Geometry check sheet. Reference: the model listing, model coordinates, mm. Give positions to 0.01 mm unless a question says otherwise; leave off trailing zeros. Loops run counter-clockwise (first coordinate to the right, second up) from the corner with the lowest first, then second, coordinate; pieces in that order, holes last.
1. Cross-section at B-B, the plane z = 0. Record the cut outline in (x, y), plus the area to 3 significant figures.
2. Cross-section at D-D, the plane z = 25.5. Record the cut outline in (x, y), plus the area to 3 significant figures.
3. Cross-section at C-C, the plane x = -55.5. Record the cut outline in (y, z).
4. Cross-section at A-A, the plane y = -1.25. Record the cut outline in (x, z).
5. Go/stop test with flat-tipped pins: pin 1 Ø1 at (y, z) = (4, 50) entering from -X; pin 2 Ø3.5 at (x, z) = (-15, 0) entering from -Y; pin 3 Ø1.5 at (y, z) = (-3.5, 36) entering from -X; pin 4 Ø1.5 at (x, y) = (-58, 2.5) entering from -Z. Record where each tip stops, or that it passes through.
6. Material ranges on L1, parallel to Z at x = 0, y = 2.5; L2, parallel to Z at x = -15, y = -0.25; L3, parallel to X at y = -3.25, z = 25, recorded low to high.
from build123d import *

# Parameters (mm, degrees)
BOSS_EXTRUDE1_DEPTH      = 5
FILLET1_R                = 7.6
M5_CLEARANCE_HOLE1_D     = 5.5
M5_CLEARANCE_HOLE1_DEPTH = 10


with BuildPart() as part:
    # Sketch1 → Boss-Extrude1 (new body, symmetric)
    with BuildSketch(Plane(origin=(0, 0, 0), x_dir=(1, 0, 0), z_dir=(0, 1, 0))):
        with BuildLine():
            Line((-15, 7.6), (15, 7.6))
            ThreePointArc((15, 7.6), (22.021484447, 2.908394086), (20.374011537, -5.374011537))
            Line((20.374011537, -5.374011537), (-54.251976926, -80))
            Line((-54.251976926, -80), (-105.748023074, -80))
            Line((-105.748023074, -80), (-20.374011537, 5.374011537))
            ThreePointArc((-20.374011537, 5.374011537), (-17.908394086, 7.021484447), (-15, 7.6))
        make_face()
    extrude(amount=BOSS_EXTRUDE1_DEPTH, both=True)

    # Fillet1
    fillet1_edges = [part.edges().sort_by_distance(p)[0] for p in [
        (-54.251976926, 0, 80),
        (-105.748023074, 0, 80),
    ]]
    fillet(fillet1_edges, radius=FILLET1_R)

    # M5 Clearance Hole1
    with Locations(Plane(origin=(0, 5, 0), x_dir=(1, 0, 0), z_dir=(0, 1, 0))):
        with Locations((-15, 0), (0, 0), (15, 0)):
            Hole(M5_CLEARANCE_HOLE1_D / 2, depth=M5_CLEARANCE_HOLE1_DEPTH)


solid = part.part
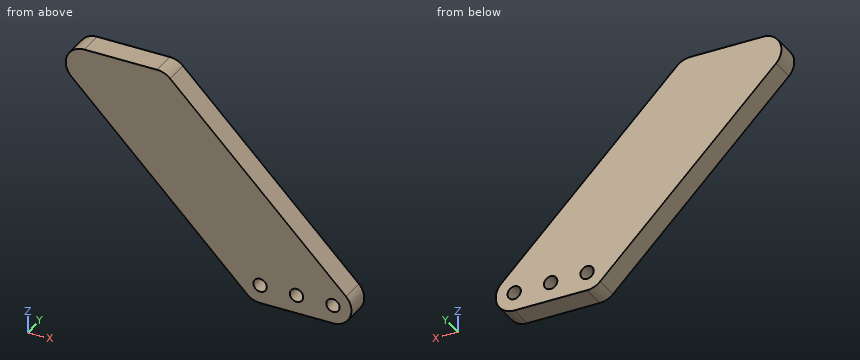
Result:
1. outline: (-25.75, -5) - (-17.75, -5) - (-17.75, 5) - (-25.75, 5) - close; (-12.25, -5) - (-2.75, -5) - (-2.75, 5) - (-12.25, 5) - close; (2.75, -5) - (12.25, -5) - (12.25, 5) - (2.75, 5) - close; (17.75, -5) - (22.6, -5) - (22.6, 5) - (17.75, 5) - close
1. area: 318 mm2
2. outline: (-51.25, -5) - (0.25, -5) - (0.25, 5) - (-51.25, 5) - close
2. area: 515 mm2
3. outline: (-5, 29.75) - (5, 29.75) - (5, 79.76) - (-5, 79.76) - close
4. outline: (-92.77, 67.03) - (-20.37, -5.37) arc R7.6 ccw to (-15, -7.6) - (15, -7.6) arc R7.6 ccw to (20.37, 5.37) - (-52.03, 77.77) arc R7.6 ccw to (-57.4, 80) - (-87.4, 80) arc R7.6 ccw to start; hole circle Ø5.5 at (-15, 0); hole circle Ø5.5 at (0, 0); hole circle Ø5.5 at (15, 0)
5. pin 1: stops at x = -76.25
5. pin 2: passes through
5. pin 3: stops at x = -62.5
5. pin 4: stops at z = 31.5
6. L1: z = -7.6 to -2.75, 2.75 to 25.75
6. L2: z = -7.6 to -2.75, 2.75 to 40.75
6. L3: x = -50.75 to 0.75
